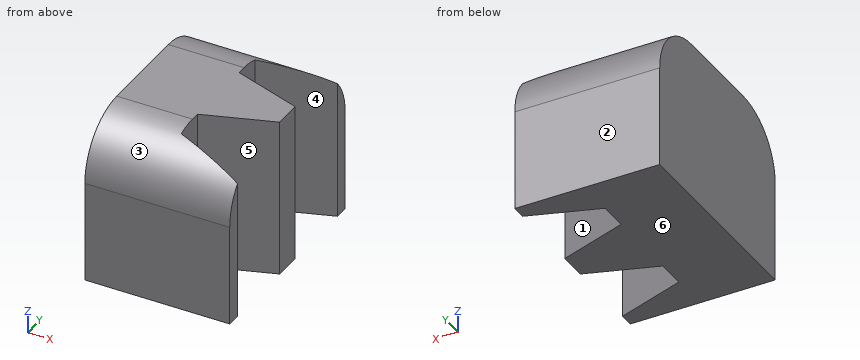
from build123d import *

# Parameters (mm, degrees)
BOSS_EXTRUDE1_DEPTH = 5.5
FILLET1_R           = 2


with BuildPart() as part:
    # Sketch1 → Boss-Extrude1 (new body)
    with BuildSketch(Plane.XY):
        Polygon((2.754977626, -3.612882911), (2.754977626, -3.127020625), (0.364622857, -2.309471144), (0.364622857, -1.303411767), (2.754977626, -0.485862286), (2.754977626, 0.485862286), (0.364622857, 1.303411767), (0.364622857, 2.309471144), (2.754977626, 3.127020625), (2.754977626, 3.612882911), (-2.245021882, 3.612882911), (-2.245021014, -3.612882911), align=None)
    extrude(amount=BOSS_EXTRUDE1_DEPTH)

    # Fillet1
    fillet1_edges = [part.edges().sort_by_distance(p)[0] for p in [
        (0.254978306, -3.612882911, 5.5),
        (0.254977872, 3.612882911, 5.5),
    ]]
    fillet(fillet1_edges, radius=FILLET1_R)


solid = part.part
Check sheet for the modelled part. Datum: model origin and axes. Units: mm. Face numbers are marked on the shaded views. A direction names the side the tool comes from. Coordinates: 2 decimals unless noted, no trailing zeros. Write each loop counter-clockwise with the first axis right and the second up, starting at its lowest first coordinate (ties: lowest second). Pieces come first, ordered by that corner, then holes. Notation, with made-up numbers: M 47,21 L 88,21 A27 cw 88,48 Z; hole C -14,24 d11. An arc over 180 degrees is marked long. Answer as CSV lines item,"result".
Q1. Mould release check, pull along Y, two halves, no side actions. Record for the marked faces 3, 4, 5 and 6: released by +Y, released by -Y, zero draft, split by the parting line, or undercut.
Check result:
face 3,"released by -Y"
face 4,"undercut"
face 5,"undercut"
face 6,"zero draft"
Q2. Cross-section at A-A (x = 0.85). Record the boundary of the cut face in (y, z), then the cut area to 3 significant figures.
Check result:
outline,"M -3.61,0 L -2.48,0 L -2.48,5.3 A2 ccw -3.61,3.5 Z; M -1.14,0 L 1.14,0 L 1.14,5.5 L -1.14,5.5 Z; M 2.48,0 L 3.61,0 L 3.61,3.5 A2 ccw 2.48,5.3 Z"
area,"23.4 mm^2"
Q3. Set-up check for the marked faces 1 and 2: record each of +Z, -Z, +X, -X, +Y, -Y from which the full face is reachable in a straight line by a thin tool's end or side.
Check result:
face 1,"+Z, -Z, +X"
face 2,"+Z, -Z, +X, -X, +Y"
Q4. Material ranges on probe 1 along Y at (x, z) = (1.15, 3.6); probe 2 along Y at (x, z) = (2.5, 2.8); probe 3 along X at (y, z) = (1.75, 4.15), recorded low to high. Write a range as from..to.
Check result:
probe 1,"-3.61..-2.58, -1.03..1.03, 2.58..3.61"
probe 2,"-3.61..-3.04, -0.57..0.57, 3.04..3.61"
probe 3,"-2.25..0.36"
Q5. Cross-section at C-C (x = -1.2). Record the boundary of the cut face in (y, z).
Check result:
outline,"M -3.61,0 L 3.61,0 L 3.61,3.5 A2 ccw 1.61,5.5 L -1.61,5.5 A2 ccw -3.61,3.5 Z"
Q6. Go/stop test with a flat-tipped pin: pin 1 (1.5 mm diameter, centred on x = 0, y = -3, fed in from +Z). Record where the tip stops, or that it passes through.
Check result:
pin 1,"z = 5.4"
Q7. Cross-section at D-D (x = 1.9). Record the boundary of the cut face in (y, z).
Check result:
outline,"M -3.61,0 L -2.83,0 L -2.83,5.08 A2 ccw -3.61,3.5 Z; M -0.78,0 L 0.78,0 L 0.78,5.5 L -0.78,5.5 Z; M 2.83,0 L 3.61,0 L 3.61,3.5 A2 ccw 2.83,5.08 Z"
Q8. Cross-section at B-B (z = 0.6). Record the boundary of the cut face in (x, y).
Check result:
outline,"M -2.25,-3.61 L 2.75,-3.61 L 2.75,-3.13 L 0.36,-2.31 L 0.36,-1.3 L 2.75,-0.49 L 2.75,0.49 L 0.36,1.3 L 0.36,2.31 L 2.75,3.13 L 2.75,3.61 L -2.25,3.61 Z"
